Check sheet for the modelled part. Datum: model origin and axes. Units: mm. A direction names the side the tool comes from. Give positions to 0.01 mm unless a question says otherwise; leave off trailing zeros. Order: outer loops, then holes, each group sorted by start corner. A loop starts at its lowest first (then second) coordinate and runs counter-clockwise, first axis right, second up.
Item 1: Material ranges on line 1 along Y through (x, z) = (32, 1799.5); line 2 along X through (y, z) = (7, 1966); line 3 along Z through (x, y) = (36, 71.5), recorded low to high.
Item 2: Release check for a two-part mould opening along X. For faces 3 (the flat face through (36, 37, 1139)), 4 (the flat face through (3.797, 40.453, 2256.907)), 5 (the flat face through (20, 75, 1114)) record: released by +X, released by -X, zero draft, split by the parting line, or undercut.
Item 3: Sectioned sample at B-B on z = 942. Record the boundary of the cut face in (x, y), and give its area (3 significant figures).
Item 4: Sectioned sample at A-A on y = 24. Record the boundary of the cut face in (x, z).
Item 5: Sectioned sample at C-C on x = 26.5. Record the boundary of the cut face in (y, z), and give its area (3 significant figures).
Item 6: Access from +Z, -Z, +X, -X, +Y, -Y to the whole of each face (thin tool, end or side, straight path). Record for faces 1 (the flat face through (4, 37, 1116)), 2 (the flat face through (40, 37, 1142)).
from build123d import *

# Parameters (mm, degrees)
F0_W     = 40
F0_H     = 75
F0_W_2   = 32
F0_H_2   = 67
F1_DEPTH = 2258.9
F3_DEPTH = 75
F5_DEPTH = 75


with BuildPart() as f1:
    # F0 (on Top) → F1 (new body)
    with BuildSketch(Plane.XY):
        with Locations((20, 37.5)):
            Rectangle(F0_W, F0_H)
        with Locations((20, 37.5)):
            Rectangle(F0_W_2, F0_H_2, mode=Mode.SUBTRACT)
    extrude(amount=F1_DEPTH)

    # F2 (on face) → F3 (cut, through all)
    with BuildSketch(Plane(origin=(0, 75, 0), x_dir=(-1, 0, 0), z_dir=(0, 1, 0))):
        Polygon((-40, 2237.899531), (0, 2258.9), (-40, 2258.9), align=None)
    extrude(amount=-F3_DEPTH, mode=Mode.SUBTRACT)

    # F4 (on face) → F5 (cut, through all)
    with BuildSketch(Plane(origin=(0, 75, 0), x_dir=(-1, 0, 0), z_dir=(0, 1, 0))):
        Polygon((-40, 0), (0, 0), (-40, 76.188773), align=None)
    extrude(amount=-F5_DEPTH, mode=Mode.SUBTRACT)


solid = f1.part
Report:
1. line 1: y = 0 to 4, 71 to 75
1. line 2: x = 0 to 4, 36 to 40
1. line 3: z = 68.57 to 2240
2. face 3: undercut
2. face 4: released by +X
2. face 5: zero draft
3. outline: (0, 0) - (40, 0) - (40, 75) - (0, 75) - close; hole (4, 4) - (36, 4) - (36, 71) - (4, 71) - close
3. area: 856 mm2
4. outline: (0, 0) - (4, 7.62) - (4, 2256.8) - (0, 2258.9) - close; (36, 68.57) - (40, 76.19) - (40, 2237.9) - (36, 2240) - close
5. outline: (0, 50.48) - (4, 50.48) - (4, 2244.99) - (0, 2244.99) - close; (71, 50.48) - (75, 50.48) - (75, 2244.99) - (71, 2244.99) - close
5. area: 17,600 mm2
6. face 1: +Z, -Z
6. face 2: +Z, -Z, +X, +Y, -Y
